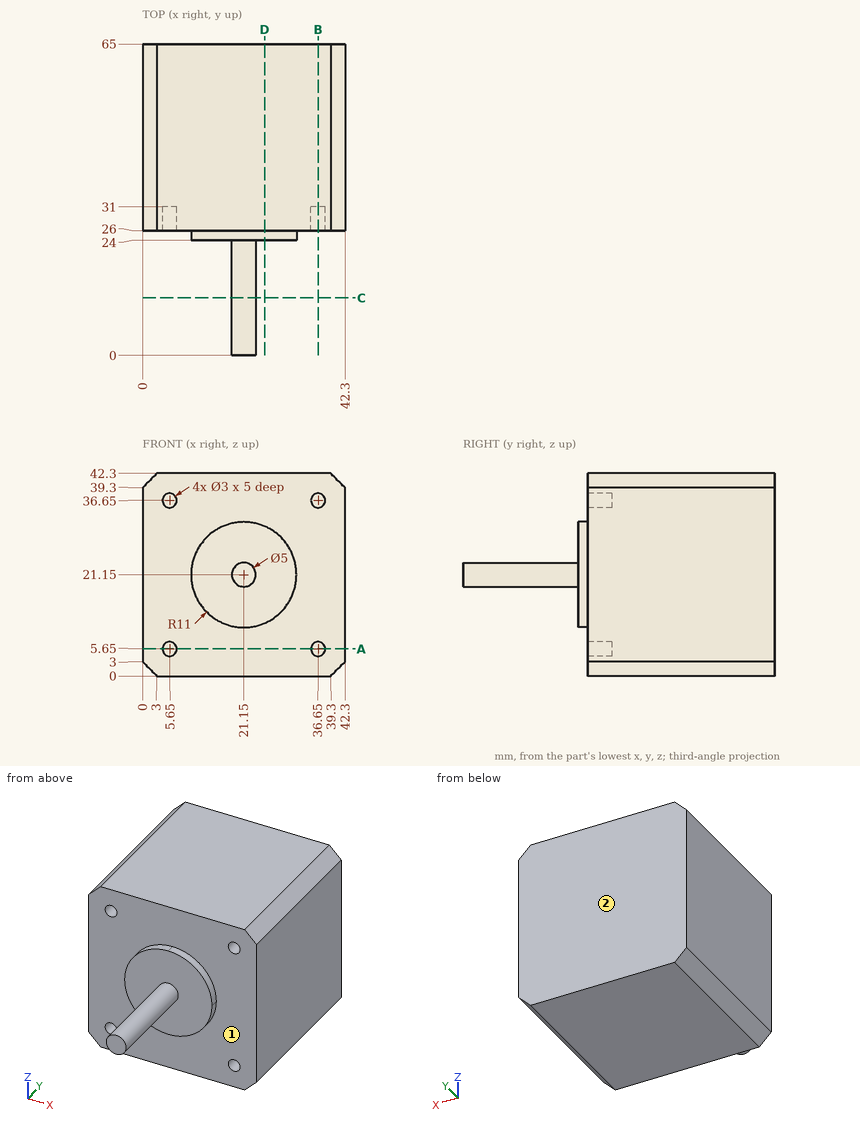
Print and shaded views of the part. All mm, measured from the part's lowest x, y and z. A direction names the side the tool comes from. Give positions to 0.01 mm unless a question says otherwise; leave off trailing zeros. Loops run counter-clockwise (first coordinate to the right, second up) from the corner with the lowest first, then second, coordinate; pieces in that order, holes last.
1) Saw through at D-D (x = 25.5). Write the cut outline in (y, z).
2) Flat gauge pins, fed straight in: pin 1 Ø3.5 at (x, z) = (5.65, 5.65) entering from -Y; pin 2 Ø1.5 at (x, z) = (36.5, 36.5) entering from -Y; pin 3 Ø1.5 at (y, z) = (23.5, 17.5) entering from +X. Where does each tip first touch, or does it go through?
3) Wall check: line 1 (Z direction, x = 36.65, y = 29.75); line 2 (Z direction, x = 36, y = 29); line 3 (Y direction, x = 17.5, z = 16.5). Give the ranges that are in metal, low to high.
4) Saw through at C-C (y = 12). Write the cut outline in (x, z), plus the area to 3 significant figures.
5) Saw through at B-B (x = 36.65). Write the cut outline in (y, z), plus the area to 3 significant figures.
6) Saw through at A-A (z = 5.65). Write the cut outline in (x, y).
7) Tool access for the marked faces 1 and 2: list every direction of +Z, -Z, +X, -X, +Y, -Y with a clear straight run to the whole face (end or side of a thin tool).
Answer block:
1. outline: (24, 11.05) - (26, 11.05) - (26, 0) - (65, 0) - (65, 42.3) - (26, 42.3) - (26, 31.25) - (24, 31.25) - close
2. pin 1: stops at y = 26
2. pin 2: stops at y = 31
2. pin 3: stops at x = 31.71
3. line 1: z = 0 to 4.15, 7.15 to 35.15, 38.15 to 42.3
3. line 2: z = 0 to 4.3, 7 to 35.3, 38 to 42.3
3. line 3: y = 24 to 65
4. outline: circle Ø5 at (21.15, 21.15)
4. area: 19.6 mm2
5. outline: (26, 0) - (65, 0) - (65, 42.3) - (26, 42.3) - (26, 38.15) - (31, 38.15) - (31, 35.15) - (26, 35.15) - (26, 7.15) - (31, 7.15) - (31, 4.15) - (26, 4.15) - close
5. area: 1,620 mm2
6. outline: (0, 26) - (4.15, 26) - (4.15, 31) - (7.15, 31) - (7.15, 26) - (35.15, 26) - (35.15, 31) - (38.15, 31) - (38.15, 26) - (42.3, 26) - (42.3, 65) - (0, 65) - close
7. face 1: -Y
7. face 2: +Z, -Z, +X, -X, +Y
